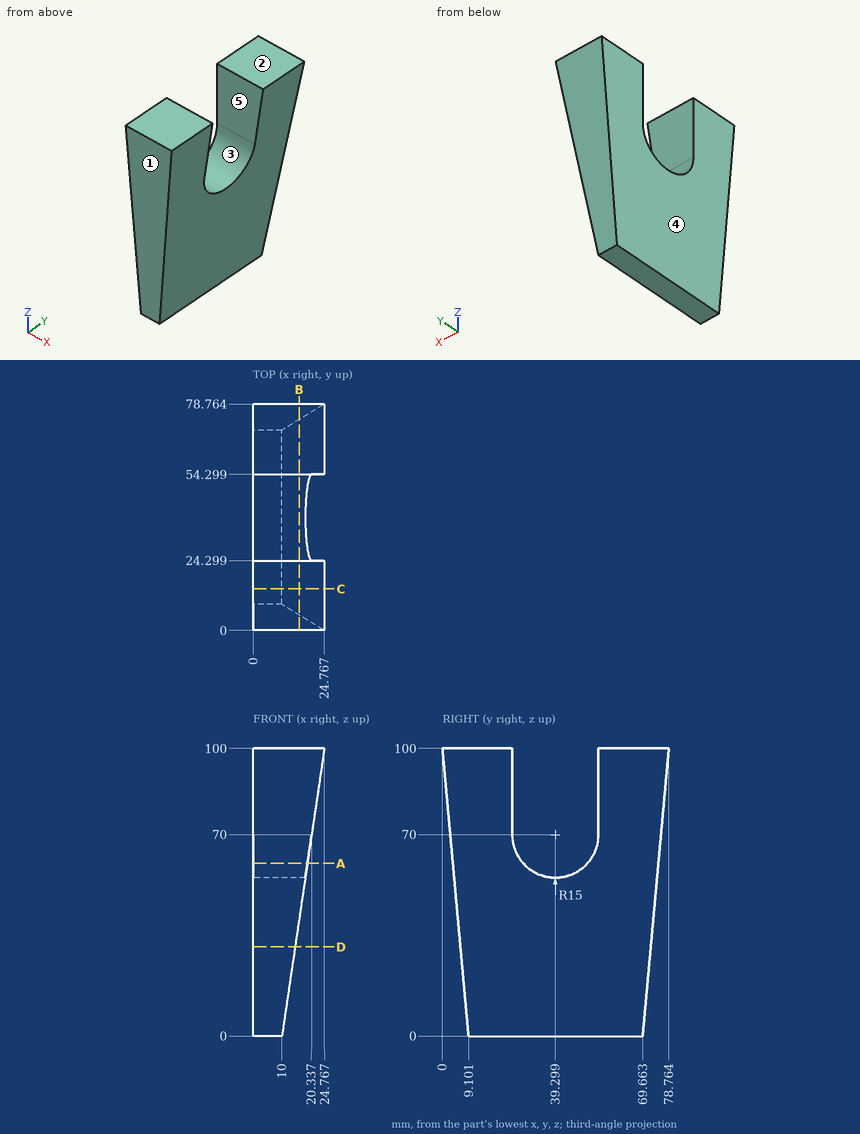
The figure shows three views and two pictorial views of one solid part (mm, origin at its lowest corner). Answer the questions. A direction names the side the tool comes from. Coordinates: 2 decimals unless noted, no trailing zeros. Write each loop counter-clockwise with the first axis right and the second up, starting at its lowest first coordinate (ties: lowest second). Pieces come first, ordered by that corner, then holes.
1. Flat-ended cylindrical pins translate along their axes: pin 1 (1 mm diameter, centred on x = 8, z = 61, fed in from -Y); pin 2 (12.5 mm diameter, centred on x = 13.5, z = 81, fed in from +Y); pin 3 (8 mm diameter, centred on x = 17, y = 29.5, fed in from +Z). Find the tip coordinate at first contact, or state that the pin passes through.
Results list:
pin 1: stops at y = 3.5
pin 2: stops at y = 77.6
pin 3: stops at z = 64.12
2. The part is cut by section D-D, the plane z = 31. Write down the section's boundary in (x, y) (1 decimal).
Results list:
outline: (0, 6.3) - (14.6, 6.3) - (14.6, 72.5) - (0, 72.5) - close
3. For the marked faces 4 and 5, determine the directions among +Z, -Z, +X, -X, +Y, -Y from which every point of the face is accessible in a straight line to the end or side of a thin tool.
Results list:
face 4: +Z, -Z, -X, +Y, -Y
face 5: +Z, +X, -X
4. Consider line 1 along Y through (x, z) = (16.5, 94) (1 decimal); line 2 along Y through (x, z) = (17, 54); line 3 along Y through (x, z) = (2.5, 54.5). Determine where each line is inside the solid, lowest interval first.
Results list:
line 1: y = 0.5 to 24.3, 54.3 to 78.2
line 2: y = 4.19 to 74.58
line 3: y = 4.14 to 74.62
5. The part is cut by section C-C, the plane y = 14.5. Write down the section's boundary in (x, z), and give its area (3 significant figures).
Results list:
outline: (0, 0) - (10, 0) - (24.77, 100) - (0, 100) - close
area: 1,740 mm2
6. For a pull along Y with two mould halves and no side action, classify the marked faces 1, 2 and 3 as +Y half, -Y half, draft (parallel to the pull), parting line (faces both ways), or undercut.
Results list:
face 1: -Y half
face 2: draft
face 3: undercut
7. The part is cut by section B-B, the plane x = 16. Write down the section's boundary in (y, z) (1 decimal), and give its area (3 significant figures).
Results list:
outline: (0, 100) - (5.4, 40.6) - (73.4, 40.6) - (78.8, 100) - (54.3, 100) - (54.3, 70) arc R15 cw to (24.3, 70) - (24.3, 100) - close
area: 3,100 mm2
8. The part is cut by section A-A, the plane z = 60. Write down the section's boundary in (x, y).
Results list:
outline: (0, 3.64) - (18.86, 3.64) - (18.86, 28.12) - (0, 28.12) - close; (0, 50.48) - (18.86, 50.48) - (18.86, 75.12) - (0, 75.12) - close
